```python
from build123d import *

# Parameters (mm, degrees)
F0_R     = 1.524
F0_R_2   = 2.38125
F0_R_3   = 2.409757
F1_DEPTH = 1.905


with BuildPart() as f1:
    # F0 (on Top) → F1 (new body)
    with BuildSketch(Plane.XY):
        Polygon((-21.506696, 26.976964), (-21.506696, 15.779537), (-21.506696, 14.255537), (-21.506696, 11.080537), (-18.331696, 11.080537), (-5.631696, 11.080537), (-2.456696, 11.080537), (-2.456696, 14.255537), (-2.456696, 14.384539), (-2.456696, 15.908539), (-2.456696, 27.062965), (-2.456696, 30.259539), (-5.653195, 30.237893), (-18.353195, 30.151892), (-21.506696, 30.130537), align=None)
        with Locations((-18.331696, 14.255537)):
            Circle(F0_R, mode=Mode.SUBTRACT)
        with Locations((-5.631696, 14.384539)):
            Circle(F0_R, mode=Mode.SUBTRACT)
        with Locations((-11.940342, 16.160537)):
            Circle(F0_R_2, mode=Mode.SUBTRACT)
        with Locations((-18.331696, 26.976964)):
            Circle(F0_R, mode=Mode.SUBTRACT)
        with Locations((-11.955501, 21.305038)):
            Circle(F0_R_3, mode=Mode.SUBTRACT)
        with Locations((-5.631696, 27.062965)):
            Circle(F0_R, mode=Mode.SUBTRACT)
    extrude(amount=F1_DEPTH)


solid = f1.part
```
The listing builds one solid part. Answer for the finished solid, in the listing's coordinates (mm). Round coordinates to 2 decimals unless told otherwise and drop trailing zeros. Loops run counter-clockwise (first coordinate to the right, second up) from the corner with the lowest first, then second, coordinate; pieces in that order, holes last. Notation, with made-up numbers: (16.5, 85) - (64.5, 85) arc R22 cw to (64.5, 108) - close; hole circle Ø4 at (47.5, -34.5). An arc over 180 degrees is marked (long way). Use one line per item in the form item = value. Start each with the question number.
1. The part is cut by section D-D on y = 15.5. Determine the outline of the cut face in (x, z) (3 decimals), then the cut area to 3 significant figures.
2. Consider line 1 (Y direction, x = -12, z = 1.05); line 2 (Y direction, x = -17.5, z = 0.15); line 3 (X direction, y = 14.75, z = 1.8). Determine where each line is inside the solid, lowest interval first. Write a range as [from, to].
3. The part is cut by section C-C on z = 1. Determine the outline of the cut face in (x, y), then the cut area to 3 significant figures.
4. The part is cut by section B-B on x = -13.5. Determine the outline of the cut face in (y, z) (3 decimals), then the cut area to 3 significant figures.
5. The part is cut by section A-A on y = 20.25. Determine the outline of the cut face in (x, z) (3 decimals), then the cut area to 3 significant figures.
6. For a pull along Y with two mould halves and no side action, classify faces 1 (the face through (-12.1, 18.7, 1.905)), 2 (the face through (-18.53, 15.767, 0.939)), 3 (the face through (-12, 11.081, 1)) as pulls with the +Y half, pulls with the -Y half, needs draft (parallel to the pull), parting line crosses it, or undercut.
7. Given pin 1 Ø5 at (x, y) = (-18.33, 14.26) entering from +Z (3 decimals); pin 2 Ø1.8 at (x, y) = (-5.63, 14.38) entering from -Z, each flat-ended and moving along its own axis, determine where each tip first touches the part or whether it passes through.
Geometry check:
q1.outline = (-21.507, 0) - (-19.211, 0) - (-19.211, 1.905) - (-21.507, 1.905) - close; (-17.452, 0) - (-14.228, 0) - (-14.228, 1.905) - (-17.452, 1.905) - close; (-9.653, 0) - (-6.67, 0) - (-6.67, 1.905) - (-9.653, 1.905) - close; (-4.593, 0) - (-2.457, 0) - (-2.457, 1.905) - (-4.593, 1.905) - close
q1.area = 20.3 mm^2
q2.line_1 = [11.08, 13.78], [18.54, 18.9], [23.71, 30.19]
q2.line_2 = [11.08, 12.98], [15.53, 25.7], [28.25, 30.16]
q2.line_3 = [-21.51, -19.77], [-16.89, -13.86], [-10.02, -7.11], [-4.15, -2.46]
q3.outline = (-21.51, 11.08) - (-2.46, 11.08) - (-2.46, 30.26) - (-21.51, 30.13) - close; hole circle Ø3.05 at (-18.33, 14.26); hole circle Ø3.05 at (-18.33, 26.98); hole circle Ø4.82 at (-11.96, 21.31); hole circle Ø4.76 at (-11.94, 16.16); hole circle Ø3.05 at (-5.63, 14.38); hole circle Ø3.05 at (-5.63, 27.06)
q3.area = 299 mm^2
q4.outline = (11.081, 0) - (14.361, 0) - (14.361, 1.905) - (11.081, 1.905) - close; (17.96, 0) - (19.455, 0) - (19.455, 1.905) - (17.96, 1.905) - close; (23.155, 0) - (30.185, 0) - (30.185, 1.905) - (23.155, 1.905) - close
q4.area = 22.5 mm^2
q5.outline = (-21.507, 0) - (-14.122, 0) - (-14.122, 1.905) - (-21.507, 1.905) - close; (-9.789, 0) - (-2.457, 0) - (-2.457, 1.905) - (-9.789, 1.905) - close
q5.area = 28.0 mm^2
q6.face_1 = needs draft
q6.face_2 = undercut
q6.face_3 = pulls with the -Y half
q7.pin_1 = 1.905
q7.pin_2 = through
